Could you check a few things on this drawing? It's one solid part, dimensions in mm from its lowest x, y, z. Give positions to 0.01 mm unless a question says otherwise; leave off trailing zeros. Order: outer loops, then holes, each group sorted by start corner. A loop starts at its lowest first (then second) coordinate and runs counter-clockwise, first axis right, second up. Notation, with made-up numbers: (-24, 48) - (24, 48) arc R21 cw to (24, 87) - close; hole circle Ø9 at (-18, 51). An arc over 180 degrees is marked (long way). Return JSON: item names as keys, results as strings.
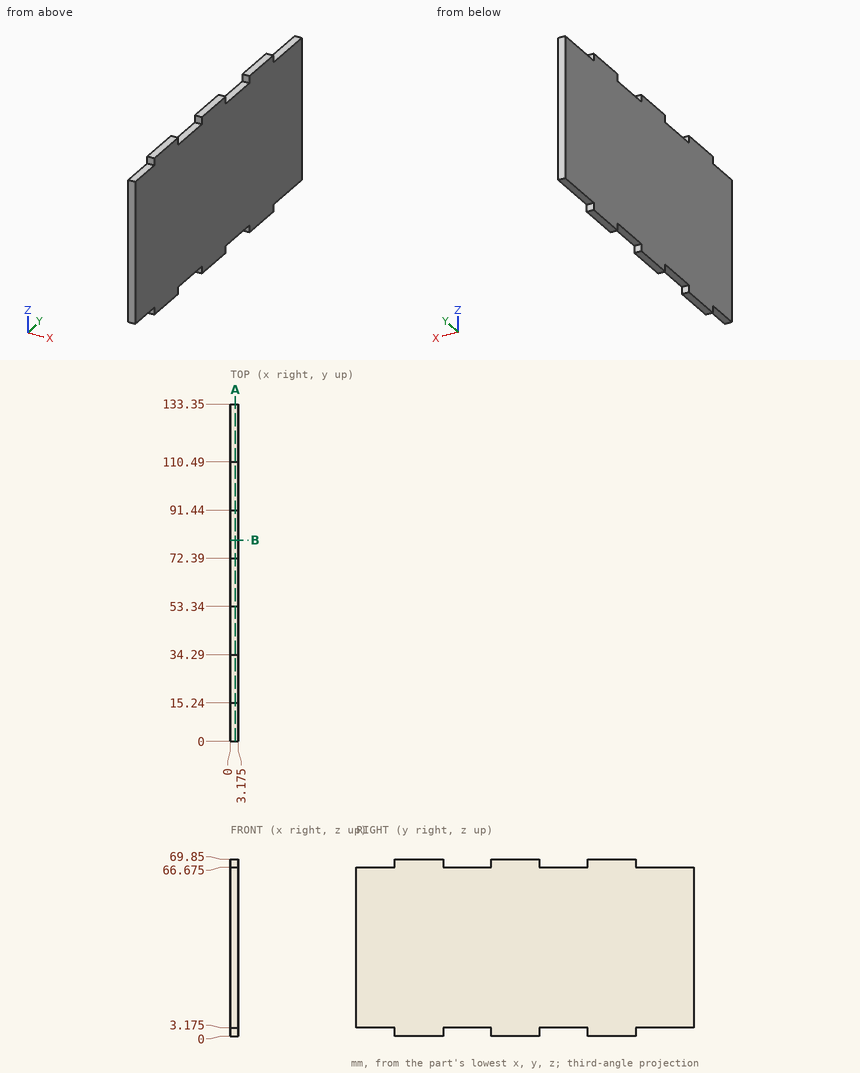
1. For pin 1 Ø1.6 at (x, y) = (1.5, 46) entering from +Z (3 decimals); pin 2 Ø1.6 at (x, y) = (1.5, 45.5) entering from -Z (3 decimals); pin 3 Ø1.6 at (x, z) = (1, 2) entering from -Y, each with a flat end and sliding along its axis, tell me the tip position at first contact or that it passes through.
Checks:
{"pin 1": "z = 66.675", "pin 2": "z = 3.175", "pin 3": "y = 15.24"}
2. Suppose I cut it at A-A (x = 2). List the corners of the cut face in (y, z) for me (3 decimals).
Checks:
{"outline": "(0, 3.175) - (15.24, 3.175) - (15.24, 0) - (34.29, 0) - (34.29, 3.175) - (53.34, 3.175) - (53.34, 0) - (72.39, 0) - (72.39, 3.175) - (91.44, 3.175) - (91.44, 0) - (110.49, 0) - (110.49, 3.175) - (133.35, 3.175) - (133.35, 66.675) - (110.49, 66.675) - (110.49, 69.85) - (91.44, 69.85) - (91.44, 66.675) - (72.39, 66.675) - (72.39, 69.85) - (53.34, 69.85) - (53.34, 66.675) - (34.29, 66.675) - (34.29, 69.85) - (15.24, 69.85) - (15.24, 66.675) - (0, 66.675) - close"}
3. If I drill on L1, parallel to Y at x = 2.7, z = 67; L2, parallel to Z at x = 2.05, y = 115.5 (3 decimals), over which ranges is the centre line in solid material (lowest first)? Write a range as [from, to].
Checks:
{"L1": "[15.24, 34.29], [53.34, 72.39], [91.44, 110.49]", "L2": "[3.175, 66.675]"}
4. Suppose I cut it at B-B (y = 79.5). List the corners of the cut face in (x, z) for me (3 decimals), plus the area to 3 significant figures.
Checks:
{"outline": "(0, 3.175) - (3.175, 3.175) - (3.175, 66.675) - (0, 66.675) - close", "area": "202 mm^2"}
